```python
from build123d import *

# Parameters (mm, degrees)
BOSS_EXTRU_1_DEPTH           = 5
ESQUISSE3_R                  = 2
ENL_V_MAT_EXTRU_1_DEPTH      = 5
ESQUISSE4_R                  = 2.75
ENL_V_MAT_EXTRU_2_DEPTH      = 1.5
ENL_V_MAT_EXTRU_3_DEPTH      = 5
ENL_V_MAT_EXTRU_3_DEPTH_BACK = 12.5
ESQUISSE5_R                  = 25.375
CONG_1_R                     = 3
CONG_2_R                     = 5
ENL_V_MAT_EXTRU_4_DEPTH      = 10
ENL_V_MAT_EXTRU_5_DEPTH      = 10


with BuildPart() as part:
    # Esquisse2 → Boss.-Extru.1 (new body)
    with BuildSketch(Plane.XY):
        with BuildLine():
            Line((-23.222436044, 101.309927053), (-23.222436044, 1.309999322))
            Line((-23.222436044, 1.309999322), (146.777563956, 1.309999322))
            Line((146.777563956, 1.309999322), (146.777563956, 101.30967935))
            add(Edge.make_bspline(
                [(146.777563956, 101.30967935), (145.378292327, 102.508699243), (143.969584716, 103.696244388), (141.124926397, 106.038205363), (139.688572163, 107.193033092), (136.777525095, 109.452247335), (135.305624265, 110.554710529), (132.312941473, 112.678620745), (130.792251165, 113.700219676), (127.677430057, 115.621696386), (126.083009921, 116.521094618), (123.612517857, 117.739485375), (122.775823394, 118.123742581), (121.071813997, 118.841506261), (120.201311014, 119.175853835), (117.565229929, 120.085558525), (115.777516182, 120.566804891), (112.144518509, 121.29157916), (110.293283793, 121.537221637), (106.597133423, 121.840020183), (104.747512209, 121.900433532), (101.046171299, 121.897761869), (99.194452085, 121.834705231), (95.489628441, 121.627070014), (93.63921765, 121.482100865), (89.947842728, 121.138535108), (88.105538062, 120.939709848), (82.585629662, 120.287230662), (78.914789341, 119.779509377), (71.58218577, 118.691503857), (67.920223281, 118.109593605), (56.945952512, 116.3014836), (49.644200811, 115.014768518), (35.051716985, 112.379241478), (27.761400742, 111.027882072), (5.899236405, 106.92561859), (-8.663476314, 104.127599978), (-23.222436044, 101.309927053)],
                knots=[0, 0, 0, 0, 0.03125, 0.03125, 0.0625, 0.0625, 0.09375, 0.09375, 0.125, 0.125, 0.15625, 0.15625, 0.171875, 0.171875, 0.1875, 0.1875, 0.21875, 0.21875, 0.25, 0.25, 0.28125, 0.28125, 0.3125, 0.3125, 0.34375, 0.34375, 0.375, 0.375, 0.4375, 0.4375, 0.5, 0.5, 0.625, 0.625, 0.75, 0.75, 1, 1, 1, 1], degree=3))
        make_face()
    extrude(amount=BOSS_EXTRU_1_DEPTH)

    # Esquisse3 → Enlèv. mat.-Extru.1 (cut)
    with BuildSketch(Plane.XY.offset(5)):
        with Locations((-18.142436044, 97.29218842)):
            Circle(ESQUISSE3_R)
        with Locations(Location((-18.142436044, 9.309999322, 0), (0, 0, 180))):
            Circle(ESQUISSE3_R)
        with Locations((141.777563956, 9.309999322)):
            Circle(ESQUISSE3_R)
        with Locations(Location((141.777563956, 97.29218842, 0), (0, 0, 180))):
            Circle(ESQUISSE3_R)
    extrude(amount=-ENL_V_MAT_EXTRU_1_DEPTH, mode=Mode.SUBTRACT)

    # Esquisse4 → Enlèv. mat.-Extru.2 (cut)
    with BuildSketch(Plane.XY.offset(5)):
        with Locations((-18.142436044, 97.29218842)):
            Circle(ESQUISSE4_R)
        with Locations((141.777563956, 97.29218842)):
            Circle(ESQUISSE4_R)
        with Locations((-18.142436044, 9.309999322)):
            Circle(ESQUISSE4_R)
        with Locations((141.777563956, 9.309999322)):
            Circle(ESQUISSE4_R)
    extrude(amount=-ENL_V_MAT_EXTRU_2_DEPTH, mode=Mode.SUBTRACT)

    # Esquisse5 → Enlèv. mat.-Extru.3 (cut, two sides: drawn at the far end of the back side and taken through both)
    with BuildSketch(Plane.XY.offset(5).offset(-ENL_V_MAT_EXTRU_3_DEPTH_BACK)):
        with Locations(Location((26.777563956, 51.309999322, 0), (0, 0, 180))):
            Circle(ESQUISSE5_R)
    extrude(amount=ENL_V_MAT_EXTRU_3_DEPTH + ENL_V_MAT_EXTRU_3_DEPTH_BACK, mode=Mode.SUBTRACT)

    # Congé1
    cong_1_edges = [part.edges().sort_by_distance(p)[0] for p in [
        (52.152563956, 51.309999322, 5),
    ]]
    fillet(cong_1_edges, radius=CONG_1_R)

    # Congé2
    cong_2_edges = [part.edges().sort_by_distance(p)[0] for p in [
        (146.777563956, 101.30967935, 2.5),
        (146.777563956, 1.309999322, 2.5),
        (-23.222436044, 1.309999322, 2.5),
        (-23.222436044, 101.309927053, 2.5),
    ]]
    fillet(cong_2_edges, radius=CONG_2_R)

    # Esquisse6 → Enlèv. mat.-Extru.4 (cut)
    with BuildSketch(Plane.XY.offset(5)):
        with BuildLine():
            Line((5.741137215, 76.376934715), (5.670426537, 76.447645393))
            ThreePointArc((5.670426537, 76.447645393), (1.639917885, 76.447645393), (1.639917885, 72.41713674))
            Line((1.639917885, 72.41713674), (1.710628563, 72.346426062))
            ThreePointArc((1.710628563, 72.346426062), (5.741137215, 72.346426062), (5.741137215, 76.376934715))
        make_face()
        with BuildLine():
            Line((47.813990696, 76.376934715), (47.884701374, 76.447645393))
            ThreePointArc((47.884701374, 76.447645393), (51.915210027, 76.447645393), (51.915210027, 72.41713674))
            Line((51.915210027, 72.41713674), (51.844499349, 72.346426062))
            ThreePointArc((51.844499349, 72.346426062), (47.813990696, 72.346426062), (47.813990696, 76.376934715))
        make_face()
        with BuildLine():
            Line((47.813990696, 26.243063929), (47.884701374, 26.172353251))
            ThreePointArc((47.884701374, 26.172353251), (51.915210027, 26.172353251), (51.915210027, 30.202861903))
            Line((51.915210027, 30.202861903), (51.844499349, 30.273572582))
            ThreePointArc((51.844499349, 30.273572582), (47.813990696, 30.273572582), (47.813990696, 26.243063929))
        make_face()
        with BuildLine():
            Line((5.741137215, 26.243063929), (5.670426537, 26.172353251))
            ThreePointArc((5.670426537, 26.172353251), (1.639917885, 26.172353251), (1.639917885, 30.202861903))
            Line((1.639917885, 30.202861903), (1.710628563, 30.273572582))
            ThreePointArc((1.710628563, 30.273572582), (5.741137215, 30.273572582), (5.741137215, 26.243063929))
        make_face()
    extrude(amount=-ENL_V_MAT_EXTRU_4_DEPTH, mode=Mode.SUBTRACT)

    # Esquisse7 → Enlèv. mat.-Extru.5 (cut)
    with BuildSketch(Plane.XY.offset(5)):
        with BuildLine():
            Line((99.027563956, 28.809999322), (104.527563956, 28.809999322))
            ThreePointArc((104.527563956, 28.809999322), (108.277563956, 25.059999322), (104.527563956, 21.309999322))
            Line((104.527563956, 21.309999322), (99.027563956, 21.309999322))
            ThreePointArc((99.027563956, 21.309999322), (95.277563956, 25.059999322), (99.027563956, 28.809999322))
        make_face()
    extrude(amount=-ENL_V_MAT_EXTRU_5_DEPTH, mode=Mode.SUBTRACT)


solid = part.part
```
Geometry: final body of the model. Coordinates: model frame, mm. A direction names the side the tool comes from. Give positions to 0.01 mm unless a question says otherwise; leave off trailing zeros. Order: outer loops, then holes, each group sorted by start corner. A loop starts at its lowest first (then second) coordinate and runs counter-clockwise, first axis right, second up. Notation, with made-up numbers: M 43.5,56 L 74.5,56 A19 ccw 74.5,73 Z; hole C -11,82.25 d5. An arc over 180 degrees is marked long. Answer as CSV lines item,"result". Start each with the question number.
1) Line query: line 1 (X direction, y = 9.31, z = 0.7); line 2 (X direction, y = 9.31, z = 4.25); line 3 (Y direction, x = 104, z = 4.25). Output: solid intervals per line, ascending. Write a range as from..to.
2) First-contact query: P1, Ø9, axis at x = -18.14, y = 97.29, coming from the +Z side; P2, Ø5, axis at x = -18.14, y = 9.31, coming from the +Z side. Flat tips, straight axial feed; report the tip coordinate or a pass-through.
3) Cut plane A-A (y = 9.31). Output: boundary loops of the cut face in (x, z), then the cut area to 4 significant figures.
4) Mould query, pull axis X, two halves, no side actions, for faces 1 (the cylindrical face through (-20.05, 8.71, 1.77)), 2 (the flat face through (-23.222, 52, 2)), 3 (the flat face through (61, 62, 0)). Classes: +X half, -X half, draft (parallel to the pull), parting line (faces both ways), or undercut.
5) Set-up query: faces 4 (the flat face through (61, 62, 5)), 5 (the cylindrical face through (108.277, 25.142, 2.535)), 6 (the cylindrical face through (-16.87, 6.87, 4.26)). Return all of +Z, -Z, +X, -X, +Y, -Y with unobstructed straight access to the full face (end or side cutting, diameter ignored); none if empty.
Findings below:
1,line 1,"x = -23.22..-20.14, -16.14..139.78, 143.78..146.78"
1,line 2,"x = -23.22..-20.89, -15.39..139.03, 144.53..146.78"
1,line 3,"y = 1.31..21.31, 28.81..121.89"
2,P1,"stops at z = 5"
2,P2,"stops at z = 3.5"
3,outline,"M -23.22,0 L -20.14,0 L -20.14,3.5 L -20.89,3.5 L -20.89,5 L -23.22,5 Z; M -16.14,0 L 139.78,0 L 139.78,3.5 L 139.03,3.5 L 139.03,5 L -15.39,5 L -15.39,3.5 L -16.14,3.5 Z; M 143.78,0 L 146.78,0 L 146.78,5 L 144.53,5 L 144.53,3.5 L 143.78,3.5 Z"
3,area,"805.5 mm²"
4,face 1,"undercut"
4,face 2,"-X half"
4,face 3,"draft"
5,face 4,"+Z, +X, -X, +Y, -Y"
5,face 5,"+Z, -Z"
5,face 6,"+Z"
